For this review, take the finished solid that the model builds, in its own axes (mm). A direction names the side the tool comes from. Coordinates: 2 decimals unless noted, no trailing zeros. Write each loop counter-clockwise with the first axis right and the second up, starting at its lowest first coordinate (ties: lowest second). Pieces come first, ordered by that corner, then holes. Notation, with made-up numbers: (52.5, -22) -> (101.5, -22) arc R23 ccw to (101.5, -13) -> close; hole circle Ø6 at (34, -32.5). An arc over 180 degrees is marked (long way). One line per item, written item: value. Start each with the question number.
1) Add section D-D (y = -7.5). State the section outline as (x, z) points.
2) Mouldability with a two-part tool opening along X and no side actions: class faces 4 (the flat face through (1, 4, 40)), 5 (the cylindrical face through (-0.219, 5.078, 20.28)), 6 (the cylindrical face through (-60, -10, 20)) as released by +X, released by -X, zero draft, split by the parting line, or undercut.
3) Machinability: for faces 1 (the flat face through (-27, -5, 20)), 2 (the cylindrical face through (48.872, -9.93, 15.386)), 3 (the flat face through (20, 5, 20)), which of the approach directions +Z, -Z, +X, -X, +Y, -Y give a long, thin tool a straight path to every point of the face, cutting with its end or side? Answer none if there is none.
4) Add section B-B (x = 0). State the section outline as (y, z) points.
5) Add section A-A (z = 20). State how many separate pieces and enclosed holes the cut face has, and give its area (3 significant figures).
6) For probe 1 along X at (y, z) = (-10.25, 20); probe 2 along Z at (x, y) = (-40, -8); probe 3 along Y at (x, z) = (25.5, 19), list the stretches that pass through material, from the lowest coordinate up. Write a range as from..to.
7) Add section C-C (y = 13.5). State the section outline as (x, z) points.
8) For pin 1 Ø12 at (x, z) = (-48, 24) entering from +Y; pin 2 Ø10 at (y, z) = (26, 35) entering from -X; pin 3 Ø3 at (x, y) = (22.5, -6.5) entering from -Z; pin 4 Ø1 at (x, z) = (47, 23) entering from -Y, all flat-tipped, find the tip position at first contact; note any pin that passes through.
Autodesk Inventor part; units mm, degrees
ref_plane "YZ Plane" through (0, 0, 0) normal (1, 0, 0) x (0, 1, 0)
ref_plane "XZ Plane" through (0, 0, 0) normal (0, 1, 0) x (-1, 0, 0)
ref_plane "XY Plane" through (0, 0, 0) normal (0, 0, 1) x (1, 0, 0)
sketch "Boceto1" plane through (0, 0, 0) normal (0, 0, 1) x (1, 0, 0)
  line L0 (-20, -15) -> (20, -15)
  line L1 (20, -15) -> (20, 15)
  line L2 (20, 15) -> (-20, 15)
  line L3 (-20, 15) -> (-20, -15)
  line L4 (-20, -15) -> (20, 15) construction
  line L5 (20, -15) -> (-20, 15) construction
  point P0 (0, 0)
  dimension "d0" = 40
  dimension "d1" = 30
extrude "Extrusión1" add sketch "Boceto1" along normal blind 40
sketch "Boceto2" plane through (0, 0, 40) normal (0, 0, 1) x (1, 0, 0)
  line L0 (20, 15) -> (-20, 15)
  circle A0 centre (0, 15) radius 10
  circle A1 centre (0, 15) radius 20
  point P0 (0, 0)
  point P1 (-10, 15)
  point P2 (10, 15)
  dimension "d4" = 20
extrude "Extrusión2" add sketch "Boceto2" against normal blind 40 contours L0 A0 A1 picked at (-3.5694, 31.1605)
sketch "Boceto3" plane through (0, 0, 40) normal (0, 0, 1) x (1, 0, 0)
  circle A0 centre (0, 15.0754) radius 10
  point P0 (0, 0)
  dimension "d7" = 20
extrude "Extrusión3" cut sketch "Boceto3" against normal blind 40
sketch "Boceto4" plane through (20, -15, 40) normal (1, 0, 0) x (0, 0, -1)
  line L0 (40, 30) -> (40, 0)
  line L1 (40, 0) -> (0, 0)
  line L2 (0, 0) -> (0, 10)
  line L3 (0, 10) -> (40, 10)
  line L4 (40, 10) -> (40, 0)
  point P0 (40, 15)
  dimension "d10" = 40
  dimension "d11" = 10
extrude "Extrusión4" add sketch "Boceto4" along normal blind 20
sketch "Boceto5" plane through (20, -5, 40) normal (0, 1, 0) x (1, 0, 0)
  line L0 (20, 40) -> (20, 0)
  circle A0 centre (20, 20) radius 10
  circle A1 centre (20, 20) radius 20
  point P0 (-20, 40)
  point P1 (20, 30)
  point P2 (20, 10)
  dimension "d14" = 20
extrude "Extrusión5" add sketch "Boceto5" against normal blind 10 contours A1 L0 A0 picked at (36.4159, 17.7748)
sketch "Boceto6" plane through (20, -5, 40) normal (0, 1, 0) x (1, 0, 0)
  line L0 (20, 10) -> (20, 30)
  circle A0 centre (20, 20) radius 10
  point P0 (-20, 40)
  dimension "d17" = 20
extrude "Extrusión6" cut sketch "Boceto6" against normal blind 10 contours A0 L0 picked at (18.4509, 17.0485)
sketch "Boceto7" plane through (-20, -15, 0) normal (-1, 0, 0) x (0, 0, 1)
  point P0 (0, 15)
sketch "Boceto8" plane through (-20, -15, 0) normal (-1, 0, 0) x (0, 0, 1)
  line L0 (0, 0) -> (40, 0)
  line L1 (0, 0) -> (40, 0)
  line L2 (40, 0) -> (40, 10)
  line L3 (40, 10) -> (0, 10)
  line L4 (0, 10) -> (0, 0)
  point P0 (0, 15)
  dimension "d20" = 40
  dimension "d21" = 10
extrude "Extrusión7" add sketch "Boceto8" along normal blind 20
sketch "Boceto9" plane through (-20, -5, 40) normal (0, 1, 0) x (1, 0, 0)
  line L0 (-20, 40) -> (-20, 0)
  circle A0 centre (-20, 20) radius 10
  circle A1 centre (-20, 20) radius 20
  point P0 (20, 40)
  point P1 (-20, 10)
  point P2 (-20, 30)
  dimension "d24" = 20
  dimension "d25" = 40
extrude "Extrusión8" add sketch "Boceto9" against normal blind 10 contours L0 A0 A1 picked at (-22.3932, 3.6239)
sketch "Boceto10" plane through (-20, -5, 40) normal (0, 1, 0) x (1, 0, 0)
  line L0 (-20, 30) -> (-20, 10)
  circle A0 centre (-20, 20) radius 10
  point P0 (20, 40)
  dimension "d28" = 20
extrude "Extrusión9" cut sketch "Boceto10" against normal blind 10 contours A0 L0 picked at (-17.3939, 17.9217)
thread "Rosca1"
thread "Rosca2"
thread "Rosca3"
thread "Rosca4"
properties part number "Tarea#1 Adrian Montalvan"
Numbers:
1. outline: (-40, 0) -> (40, 0) arc R20 ccw to (40, 40) -> (-40, 40) arc R20 ccw to start; hole circle Ø20 at (-40, 20); hole circle Ø20 at (40, 20)
2. face 4: zero draft
2. face 5: undercut
2. face 6: released by -X
3. face 1: +Z, -Z, -X, +Y
3. face 2: +Y, -Y
3. face 3: +Z, -Z, +X, +Y
4. outline: (-15, 0) -> (5.08, 0) -> (5.08, 40) -> (-15, 40) -> close; (25.08, 0) -> (35, 0) -> (35, 40) -> (25.08, 40) -> close
5. separate pieces: 3
5. enclosed holes: 1
5. area: 1,910 mm²
6. probe 1: -60..-50, -30..30, 50..60
6. probe 2: 0..10, 30..40
6. probe 3: -15..-5
7. outline: (-20, 0) -> (-9.88, 0) -> (-9.88, 40) -> (-20, 40) -> close; (9.88, 0) -> (20, 0) -> (20, 40) -> (9.88, 40) -> close
8. pin 1: y = -5
8. pin 2: x = -19.08
8. pin 3: z = 0
8. pin 4: through
